Check sheet for the modelled part. Datum: model origin and axes. Units: mm. Coordinates: 2 decimals unless noted, no trailing zeros. Write each loop counter-clockwise with the first axis right and the second up, starting at its lowest first coordinate (ties: lowest second). Pieces come first, ordered by that corner, then holes. Notation, with made-up numbers: (58.25, 81.5) -> (91.25, 81.5) arc R33 ccw to (91.25, 120.5) -> close; hole circle Ø9 at (17, -29). An arc over 180 degrees is marked (long way). Put each result on its own line as item: value.
Autodesk Inventor part; units mm, degrees
ref_plane "YZ Plane" through (0, 0, 0) normal (1, 0, 0) x (0, 1, 0)
ref_plane "XZ Plane" through (0, 0, 0) normal (0, 1, 0) x (-1, 0, 0)
ref_plane "XY Plane" through (0, 0, 0) normal (0, 0, 1) x (1, 0, 0)
sketch "Sketch1" plane through (0, 0, 0) normal (0, 0, 1) x (1, 0, 0)
  arc A0 (22.5, -67.5) -> (27.5, -62.5) centre (22.5, -62.5) ccw
  line L0 (27.5, 62.5) -> (27.5, -62.5)
  arc A1 (27.5, 62.5) -> (22.5, 67.5) centre (22.5, 62.5) ccw
  line L1 (-22.5, 67.5) -> (22.5, 67.5)
  arc A2 (-22.5, 67.5) -> (-27.5, 62.5) centre (-22.5, 62.5) ccw
  line L2 (-27.5, -62.5) -> (-27.5, 62.5)
  arc A3 (-27.5, -62.5) -> (-22.5, -67.5) centre (-22.5, -62.5) ccw
  line L3 (22.5, -67.5) -> (-22.5, -67.5)
  circle A4 centre (20.5, -60.5) radius 1.5 construction
  circle A5 centre (20.5, 60.5) radius 1.5 construction
  circle A6 centre (-20.5, 60.5) radius 1.5 construction
  circle A7 centre (-20.5, -60.5) radius 1.5 construction
extrude "Extrusion1" add sketch "Sketch1" against normal blind 3
sketch "Sketch4" plane through (0, 0, -3) normal (0, 0, -1) x (-1, 0, 0)
  point P0 (0, 0)
  point P1 (20.5, -60.5)
  point P2 (-20.5, -60.5)
  point P3 (20.5, 60.5)
  point P4 (-20.5, 60.5)
hole "Hole1" at (-20.5, -60.5, -3) at (20.5, -60.5, -3) at (-20.5, 60.5, -3) at (20.5, 60.5, -3) direction (0, 0, 1) diameter 3 end through all countersink diameter 6.2 countersink angle 90
equation "\"d3\" = Plate_thickness"
equation "\"Plate_thickness\" = 3"
equation "\"Top_Plate_Bottom_to_PowerPcb_Bottom\" = 2.7"
properties part number "Box_Bottom_Plate" material "Aluminum 6061"
Q1. Material ranges on line 1 along Y through (x, z) = (20.5, -0.35); line 2 along X through (y, z) = (-60.5, -0.4); line 3 along Y through (x, z) = (-19.5, -1.85), recorded low to high.
Recorded:
line 1: y = -67.5 to -62, -59 to 59, 62 to 67.5
line 2: x = -27.5 to -22, -19 to 19, 22 to 27.5
line 3: y = -67.5 to -62.17, -58.83 to 58.83, 62.17 to 67.5
Q2. Depth check by flat-ended pin: P1, Ø5, axis at x = 20.5, y = 60.5, coming from the -Z side. Enter the tip coordinate at first touch or a pass-through.
Recorded:
P1: stops at z = -2.4
Q3. Cross-section at B-B (x = 20.5). Record the cut outline in (y, z), plus the area to 3 significant figures.
Recorded:
outline: (-67.5, -3) -> (-63.6, -3) -> (-62, -1.4) -> (-62, 0) -> (-67.5, 0) -> close; (-59, -1.4) -> (-57.4, -3) -> (57.4, -3) -> (59, -1.4) -> (59, 0) -> (-59, 0) -> close; (62, -1.4) -> (63.6, -3) -> (67.5, -3) -> (67.5, 0) -> (62, 0) -> close
area: 382 mm2
Q4. Cross-section at A-A (y = 60.5). Record the cut outline in (x, z), plus the area to 3 significant figures.
Recorded:
outline: (-27.5, -3) -> (-23.6, -3) -> (-22, -1.4) -> (-22, 0) -> (-27.5, 0) -> close; (-19, -1.4) -> (-17.4, -3) -> (17.4, -3) -> (19, -1.4) -> (19, 0) -> (-19, 0) -> close; (22, -1.4) -> (23.6, -3) -> (27.5, -3) -> (27.5, 0) -> (22, 0) -> close
area: 142 mm2
Q5. Mould release check, pull along Y, two halves, no side actions. Record for faces 1 (the cylindrical face through (-26.07, -66, -1.48)), 2 (the flat face through (0, 1, 0)), 3 (the cylindrical face through (-20.95, -59.07, -0.69)): released by +Y, released by -Y, zero draft, split by the parting line, or undercut.
Recorded:
face 1: released by -Y
face 2: zero draft
face 3: undercut
